Autodesk Fusion 360 part; units mm, degrees
sketch "Esboço1" plane through (0, 0, 0) normal (0, 1, 0) x (1, 0, 0)
  line L0 (-74.1987, -2.4172) -> (-64.1987, -2.4172)
  line L1 (-64.1987, -2.4172) -> (-64.1987, -17.4172)
  line L2 (-64.1987, -17.4172) -> (-49.1987, -17.4172)
  line L3 (-49.1987, -17.4172) -> (-49.1987, -1)
  line L4 (-49.1987, -1) -> (-49.1987, -2.4172)
  line L5 (-49.1987, -2.4172) -> (-39.1987, -2.4172)
  line L6 (-39.1987, -2.4172) -> (-39.1987, -7.4172)
  line L7 (-74.1987, -2.4172) -> (-74.1987, -7.4172)
  line L8 (-74.1987, -7.4172) -> (-66.6987, -7.4172)
  line L9 (-66.6987, -7.4172) -> (-66.6987, -16.9172)
  line L10 (-39.1987, -7.4172) -> (-46.6987, -7.4172)
  line L11 (-46.6987, -7.4172) -> (-46.6987, -16.9172)
  line L12 (-63.6987, -19.9172) -> (-49.6987, -19.9172)
  arc A0 (-66.6987, -16.9172) -> (-63.6987, -19.9172) centre (-63.6987, -16.9172) ccw
  arc A1 (-49.6987, -19.9172) -> (-46.6987, -16.9172) centre (-49.6987, -16.9172) ccw
  point P0 (-66.6987, -19.9172)
  point P1 (-46.6987, -19.9172)
  dimension "d1" = 10
  dimension "d2" = 15
  dimension "d3" = 15
  dimension "d4" = 10
  dimension "d5" = 5
  dimension "d6" = 5
  dimension "d7" = 7.5
  dimension "d8" = 12.5
  dimension "d9" = 7.5
  dimension "d10" = 12.5
  dimension "d11" = 3
extrude "Extrusão1" add sketch "Esboço1" along normal blind 25
sketch "Esboço2" plane through (0, 0, 0) normal (0, 0, 1) x (1, 0, 0)
hole "Furo1" at (-70.4487, 12.5, 7.4172) direction (0, 0, -1) diameter 2.5 depth 9 tip angle 118
hole "Furo2" at (-42.9487, 12.5, 7.4172) direction (0, 0, -1) diameter 2.5 depth 9 tip angle 118
Geometry check sheet. Reference: the model listing, model coordinates, mm. A direction names the side the tool comes from. Round coordinates to 2 decimals unless told otherwise and drop trailing zeros. Order: outer loops, then holes, each group sorted by start corner. A loop starts at its lowest first (then second) coordinate and runs counter-clockwise, first axis right, second up. Notation, with made-up numbers: (46, 29.25) - (62, 29.25) arc R20 cw to (62, 42.25) - close; hole circle Ø7 at (37, 44). An arc over 180 degrees is marked (long way). Use a Markdown table: item, result. Add a question column.
(1) Depth check by flat-ended pin: pin 1 (1.5 mm diameter, centred on y = 15.5, z = 16.5, fed in from +X); pin 2 (6 mm diameter, centred on x = -42, y = 13.5, fed in from +Z); pin 3 (5 mm diameter, centred on y = 13, z = 11, fed in from -X). Enter the tip coordinate at first touch or a pass-through.
(2) Tool access check on faces 4 (the flat face through (-64.199, 12, 10)), 5 (the flat face through (-39.199, 12, 5)), 6 (the flat face through (-41, 12, 7.417)), 7 (the cylindrical face through (-41.73, 12.77, 4.88)), 8 (the flat face through (-66.699, 12, 12)). Record the directions out of +Z, -Z, +X, -X, +Y, -Y that give a thin tool (end or side, any length) a straight path to the whole face; none if there is none.
(3) Sectioned sample at B-B, the plane y = 4.75. Enter the section's corners in (x, z), and give its area (3 significant figures).
(4) Material ranges on line 1 along X through (y, z) = (12.5, 4.05); line 2 along X through (y, z) = (23.5, 5.25); line 3 along X through (y, z) = (19.75, 14.25), recorded low to high. Write a range as [from, to].
(5) Release check for a two-part mould opening along X. For faces 1 (the flat face through (-49, 25, 9)), 2 (the cylindrical face through (-65.8, 12.32, 19.06)), 3 (the cylindrical face through (-71.69, 12.66, 4.88)) record: pulls with the +X half, pulls with the -X half, needs draft (parallel to the pull), parting line crosses it, or undercut.
(6) Sectioned sample at A-A, the plane y = 12.5. Enter the section's corners in (x, z).
(7) Sectioned sample at C-C, the plane x = -59. Enter the section's corners in (y, z), and give its area (3 significant figures).
(8) Sectioned sample at D-D, the plane z = 18. Enter the section's corners in (x, y).
Answers below:
| question | item | result |
|---|---|---|
| 1 | pin 1 | x = -46.7 |
| 1 | pin 2 | z = 7.42 |
| 1 | pin 3 | x = -66.7 |
| 2 | face 4 | -Z, +Y, -Y |
| 2 | face 5 | +Z, -Z, +X, +Y, -Y |
| 2 | face 6 | +Z, +X, +Y, -Y |
| 2 | face 7 | +Z, -Z |
| 2 | face 8 | +Z, -X, +Y, -Y |
| 3 | outline | (-74.2, 2.42) - (-64.2, 2.42) - (-64.2, 17.42) - (-49.2, 17.42) - (-49.2, 2.42) - (-39.2, 2.42) - (-39.2, 7.42) - (-46.7, 7.42) - (-46.7, 16.92) arc R3 ccw to (-49.7, 19.92) - (-63.7, 19.92) arc R3 ccw to (-66.7, 16.92) - (-66.7, 7.42) - (-74.2, 7.42) - close |
| 3 | area | 196 mm² |
| 4 | line 1 | [-74.2, -71.7], [-69.2, -64.2], [-49.2, -44.2], [-41.7, -39.2] |
| 4 | line 2 | [-74.2, -64.2], [-49.2, -39.2] |
| 4 | line 3 | [-66.7, -64.2], [-49.2, -46.7] |
| 5 | face 1 | needs draft |
| 5 | face 2 | pulls with the -X half |
| 5 | face 3 | undercut |
| 6 | outline | (-74.2, 2.42) - (-71.7, 2.42) - (-71.7, 7.42) - (-74.2, 7.42) - close; (-69.2, 2.42) - (-64.2, 2.42) - (-64.2, 17.42) - (-49.2, 17.42) - (-49.2, 2.42) - (-44.2, 2.42) - (-44.2, 7.42) - (-46.7, 7.42) - (-46.7, 16.92) arc R3 ccw to (-49.7, 19.92) - (-63.7, 19.92) arc R3 ccw to (-66.7, 16.92) - (-66.7, 7.42) - (-69.2, 7.42) - close; (-41.7, 2.42) - (-39.2, 2.42) - (-39.2, 7.42) - (-41.7, 7.42) - close |
| 7 | outline | (0, 17.42) - (25, 17.42) - (25, 19.92) - (0, 19.92) - close |
| 7 | area | 62.5 mm² |
| 8 | outline | (-66.5, 0) - (-46.9, 0) - (-46.9, 25) - (-66.5, 25) - close |
